Could you check a few things on this model? Use its own coordinates, in mm. A direction names the side the tool comes from. Give positions to 0.01 mm unless a question says otherwise; leave off trailing zeros. Order: outer loops, then holes, each group sorted by start corner. A loop starts at its lowest first (then second) coordinate and runs counter-clockwise, first axis right, second up. Notation, with made-up numbers: M 73,39 L 106,39 A14 ccw 106,48 Z; hole C 55.5,5.5 d7. An arc over 180 degrees is marked long. Use a Markdown table: item, result. Add a question column.
Solid Edge part; units mm, degrees
sketch "Sketch1" plane through (0, 0, 0) normal (0, 0, 1) x (1, 0, 0)
  circle A0 centre (0, 0) radius 1.425
extrude "Protrusion1" add sketch "Sketch1" against normal blind 8
sketch "Sketch2" plane through (0, 0, 0) normal (0, 0, 1) x (1, 0, 0)
  circle A0 centre (0, 0) radius 2.75
extrude "ExtrudedProtrusion_2" add sketch "Sketch2" along normal blind 2
sketch "Sketch3" plane through (0, 0, 2) normal (0, 0, 1) x (1, 0, 0)
  line L0 (3.6964, 0.4) -> (-3.6964, 0.4)
  line L1 (-3.6964, 0.4) -> (-3.6964, -0.4)
  line L2 (-3.6964, -0.4) -> (3.6964, -0.4)
  line L3 (3.6964, -0.4) -> (3.6964, 0.4)
extrude "ExtrudedCutout_1" cut sketch "Sketch3" against normal blind 0.5
properties material "Graphite"
1) Please list where these lines run through material, in increasing order: line 1 (Z direction, x = 1.8, y = -1.75); line 2 (Y direction, x = 0.85, z = 1.75); line 3 (Z direction, x = 2.45, y = -0.3). Write a range as from..to.
2) For pin 1 (1.5 mm diameter, centred on x = 0, z = -5.5, fed in from -Y) (3 decimals); pin 2 (3 mm diameter, centred on y = 0, z = -6.5, fed in from +X) (3 decimals); pin 3 (2 mm diameter, centred on y = -2, z = -5, fed in from +X), each with a flat end and sliding along its axis, tell me the tip position at first contact or that it passes through.
3) Suppose I cut it at A-A on y = 0. Please give me the cut outline in (x, z) (3 decimals).
4) For faces 1 (the face through (1.2, -1.2, 0)), 2 (the face through (0, -1, 2)), which set-ups out of +Z, -Z, +X, -X, +Y, -Y let a thin tool reach every point of the face, with its end or its side?
5) Suppose I cut it at C-C on z = -3.5. Please give me the cut outline in (x, y) (3 decimals), and give its area (3 significant figures).
6) Suppose I cut it at D-D on y = 0.85. Please give me the cut outline in (x, z).
7) Suppose I cut it at B-B on x = 0. Please give me the cut outline in (y, z) (3 decimals), and give its area (3 significant figures).
Values found:
| question | item | result |
|---|---|---|
| 1 | line 1 | z = 0..2 |
| 1 | line 2 | y = -2.62..-0.4, 0.4..2.62 |
| 1 | line 3 | z = 0..1.5 |
| 2 | pin 1 | stops at y = -1.425 |
| 2 | pin 2 | stops at x = 1.425 |
| 2 | pin 3 | stops at x = 1.02 |
| 3 | outline | M -2.75,0 L -1.425,0 L -1.425,-8 L 1.425,-8 L 1.425,0 L 2.75,0 L 2.75,1.5 L -2.75,1.5 Z |
| 4 | face 1 | -Z |
| 4 | face 2 | +Z, +X, -X, +Y, -Y |
| 5 | outline | C 0,0 d2.85 |
| 5 | area | 6.38 mm^2 |
| 6 | outline | M -2.62,0 L -1.14,0 L -1.14,-8 L 1.14,-8 L 1.14,0 L 2.62,0 L 2.62,2 L -2.62,2 Z |
| 7 | outline | M -2.75,0 L -1.425,0 L -1.425,-8 L 1.425,-8 L 1.425,0 L 2.75,0 L 2.75,2 L 0.4,2 L 0.4,1.5 L -0.4,1.5 L -0.4,2 L -2.75,2 Z |
| 7 | area | 33.4 mm^2 |
